For this review, take the finished solid that the model builds, in its own axes (mm). A direction names the side the tool comes from. Give positions to 0.01 mm unless a question says otherwise; leave off trailing zeros. Loops run counter-clockwise (first coordinate to the right, second up) from the corner with the lowest first, then second, coordinate; pieces in that order, holes last. Notation, with made-up numbers: M 0.25,10 L 46.25,10 A16 ccw 46.25,27 Z; hole C 78,-33.75 d1. An arc over 180 degrees is marked long. Use CSV: the item, a comma, the result in double quotes. Start each with the question number.
1. Insertion check: P1, Ø5, axis at x = 96, z = 30, coming from the -Y side; P2, Ø12, axis at x = 48, z = -21, coming from the +Y side; P3, Ø12, axis at x = 30.5, z = 0, coming from the -Y side; P4, Ø10, axis at x = 89.5, z = 4.5, coming from the +Y side. Each pin has a flat end and moves straight along its axis. Give the tip position at first contact, or say it passes through.
2. To check wall thickness, follow line 1 (Z direction, x = 83.5, y = 0); line 2 (X direction, y = 10.5, z = 12.5); line 3 (X direction, y = 34.5, z = -35.5). State the ranges of each line that lie inside material, in increasing order. Write a range as [from, to].
3. Take a section at A-A, the plane x = 41. Write out the cut boundary in (y, z).
4. Tool access review of faces 1 (the face through (64.908, -4.435, 33.776)), 2 (the face through (0, -1, 1)): name each direction out of +Z, -Z, +X, -X, +Y, -Y from which nothing blocks a thin tool from reaching the whole face with its end or side.
from build123d import *


with BuildPart() as part:
    # Sketch1 → Revolve5 (revolve)
    with BuildSketch(Plane.XY):
        with BuildLine():
            Line((0, 0), (120.65, 0))
            Line((120.65, 0), (115.974515988, 16.285996254))
            Line((115.974515988, 16.285996254), (109.624515988, 16.285996254))
            Line((109.624515988, 16.285996254), (109.624515988, 25.175996254))
            Line((109.624515988, 25.175996254), (93.114515988, 25.175996254))
            ThreePointArc((93.114515988, 25.175996254), (90.510695272, 31.462175539), (84.224515988, 34.065996254))
            Line((84.224515988, 34.065996254), (46.124515988, 34.065996254))
            ThreePointArc((46.124515988, 34.065996254), (39.838336703, 36.66981697), (37.234515988, 42.955996254))
            Line((37.234515988, 42.955996254), (28.344515988, 42.955996254))
            Line((28.344515988, 42.955996254), (12.7, 49.53))
            Line((12.7, 49.53), (0, 49.53))
            Line((0, 49.53), (0, 0))
        make_face()
    revolve(axis=Axis((0, 0, 0), (1, 0, 0)))


solid = part.part
Result set:
1,P1,"through"
1,P2,"y = 30.59"
1,P3,"y = -44.57"
1,P4,"y = 33.96"
2,line 1,"[-34.07, 34.07]"
2,line 2,"[0, 109.62]"
2,line 3,"[0, 12.77]"
3,outline,"C 0,0 d71.38"
4,face 1,"+X"
4,face 2,"+Z, -Z, -X, +Y, -Y"
